The model under review builds one solid part; all positions refer to its coordinate system, in mm. Coordinates: 2 decimals unless noted, no trailing zeros. Write each loop counter-clockwise with the first axis right and the second up, starting at its lowest first coordinate (ties: lowest second). Pieces come first, ordered by that corner, then holes. Notation, with made-up numbers: (40, 52) - (75, 52) arc R31 cw to (75, 85) - close; hole circle Ø5 at (76, -15.5). An arc over 180 degrees is marked (long way). Put each result on its own line as item: value.
from build123d import *

# Parameters (mm, degrees)
SKETCH1_W                         = 127
SKETCH1_H                         = 177.8
BOSS_EXTRUDE1_DEPTH               = 4.7625
F_10_CLEARANCE_HOLE1_D            = 5.1054
TAPPED_HOLE_FOR_10_32_HELICOIL1_D = 5.1054
TAPPED_HOLE_FOR_10_32_HELICOIL2_D = 5.1054
F_4_40_TAPPED_HOLE1_D             = 2.2606


with BuildPart() as part:
    # Sketch1 → Boss-Extrude1 (new, symmetric)
    with BuildSketch(Plane.XY):
        Rectangle(SKETCH1_W, SKETCH1_H)
    extrude(amount=BOSS_EXTRUDE1_DEPTH, both=True)

    # #10 Clearance Hole1 (through all)
    with Locations(Plane(origin=(0, 0, -4.7625), x_dir=(-1, 0, 0), z_dir=(0, 0, -1))):
        with Locations((-57.15, 82.55), (57.15, 82.55), (57.15, -82.55), (-57.15, -82.55)):
            Hole(F_10_CLEARANCE_HOLE1_D / 2)

    # Tapped Hole for #10-32 Helicoil1 (through all)
    with Locations(Plane(origin=(0, 0, -4.7625), x_dir=(-1, 0, 0), z_dir=(0, 0, -1))):
        with Locations((-15.875, 71.4375), (15.875, 11.1125), (-15.875, 11.1125), (15.875, 71.4375), (-15.875, -11.1125), (15.875, -71.4375), (-15.875, -71.4375), (15.875, -11.1125)):
            Hole(TAPPED_HOLE_FOR_10_32_HELICOIL1_D / 2)

    # Tapped Hole for #10-32 Helicoil2 (through all)
    with Locations(Plane(origin=(0, 0, -4.7625), x_dir=(-1, 0, 0), z_dir=(0, 0, -1))):
        with Locations((-42.06875, 19.05), (-42.06875, -19.05)):
            Hole(TAPPED_HOLE_FOR_10_32_HELICOIL2_D / 2)

    # #4-40 Tapped Hole1 (through all)
    with Locations(Plane.XY.offset(4.7625)):
        with Locations((-20.701, 67.1195), (-42.799, 56.7055), (-20.701, -21.082), (-42.799, -10.668)):
            Hole(F_4_40_TAPPED_HOLE1_D / 2)


solid = part.part
1. Consider section A-A on x = -57.15. State the section outline as (y, z) points, plus the area to 3 significant figures.
Determined:
outline: (-88.9, -4.76) - (-85.1, -4.76) - (-85.1, 4.76) - (-88.9, 4.76) - close; (-80, -4.76) - (80, -4.76) - (80, 4.76) - (-80, 4.76) - close; (85.1, -4.76) - (88.9, -4.76) - (88.9, 4.76) - (85.1, 4.76) - close
area: 1,600 mm^2
2. To check wall thickness, follow probe 1 along Y at (x, z) = (-16, -4); probe 2 along Y at (x, z) = (57.15, 2); probe 3 along Y at (x, z) = (-42, 3.5). State the ranges of each line that lie inside material, in increasing order.
Determined:
probe 1: y = -88.9 to -73.99, -68.89 to -13.66, -8.56 to 8.56, 13.66 to 68.89, 73.99 to 88.9
probe 2: y = -88.9 to -85.1, -80 to 80, 85.1 to 88.9
probe 3: y = -88.9 to -11.47, -9.87 to 55.91, 57.5 to 88.9
3. The part is to be moulded in two halves that separate along X. For faces 1 (the flat face through (-1, 1, -4.762)), 2 (the flat face through (-63.5, -1, 0)), 3 (the cylindrical face through (54.6, 82.7, 0.1)), say which applies: +X half, -X half, draft (parallel to the pull), parting line (faces both ways), or undercut.
Determined:
face 1: draft
face 2: -X half
face 3: undercut
4. Consider section B-B on y = -82.55. State the section outline as (x, z) points.
Determined:
outline: (-63.5, -4.76) - (-59.7, -4.76) - (-59.7, 4.76) - (-63.5, 4.76) - close; (-54.6, -4.76) - (54.6, -4.76) - (54.6, 4.76) - (-54.6, 4.76) - close; (59.7, -4.76) - (63.5, -4.76) - (63.5, 4.76) - (59.7, 4.76) - close
5. Consider section C-C on y = 19.05. State the section outline as (x, z) points.
Determined:
outline: (-63.5, -4.76) - (39.52, -4.76) - (39.52, 4.76) - (-63.5, 4.76) - close; (44.62, -4.76) - (63.5, -4.76) - (63.5, 4.76) - (44.62, 4.76) - close
6. For pin 1 Ø3 at (x, y) = (-42.799, -10.668) entering from +Z, flat-tipped, find the tip position at first contact; note if it passes through.
Determined:
pin 1: stops at z = 4.76
